Here's how the part is built. I have some questions about the finished solid (model axes, mm). A direction names the side the tool comes from. Coordinates: 2 decimals unless noted, no trailing zeros. Write each loop counter-clockwise with the first axis right and the second up, starting at its lowest first coordinate (ties: lowest second). Pieces come first, ordered by that corner, then holes.
```python
from build123d import *

# Parameters (mm, degrees)
SKETCH1_R           = 4.25
BOSS_EXTRUDE1_DEPTH = 20
SKETCH3_R           = 3.55
CUT_EXTRUDE2_DEPTH  = 10.5
SKETCH2_R           = 3.2
CUT_EXTRUDE3_DEPTH  = 10.5


with BuildPart() as part:
    # Sketch1 → Boss-Extrude1 (new body)
    with BuildSketch(Plane(origin=(0, 0, 0), x_dir=(1, 0, 0), z_dir=(0, 1, 0))):
        Polygon((0, 0), (0, 50), (57.5, 50), (72.5, 30), (87.5, 50), (145, 50), (145, 0), align=None)
        with Locations(Location((15, 20.25, 0), (0, 0, 270))):
            Circle(SKETCH1_R, mode=Mode.SUBTRACT)
        with Locations(Location((72.5, 14.25, 0), (0, 0, 270))):
            Circle(SKETCH1_R, mode=Mode.SUBTRACT)
        with Locations(Location((130, 20.25, 0), (0, 0, 270))):
            Circle(SKETCH1_R, mode=Mode.SUBTRACT)
    extrude(amount=BOSS_EXTRUDE1_DEPTH)

    # Sketch3 → Cut-Extrude2 (cut)
    with BuildSketch(Plane.XY):
        with Locations((25, 10)):
            Circle(SKETCH3_R)
        with Locations((120, 10)):
            Circle(SKETCH3_R)
    extrude(amount=-CUT_EXTRUDE2_DEPTH, mode=Mode.SUBTRACT)

    # Sketch2 → Cut-Extrude3 (cut)
    with BuildSketch(Plane(origin=(0, 20, 0), x_dir=(1, 0, 0), z_dir=(0, 1, 0))):
        with Locations(Location((22.5, 35, 0), (0, 0, 270))):
            Circle(SKETCH2_R)
        with Locations(Location((122.5, 35, 0), (0, 0, 270))):
            Circle(SKETCH2_R)
    extrude(amount=-CUT_EXTRUDE3_DEPTH, mode=Mode.SUBTRACT)


solid = part.part
```
1) Imagine slicing it at C-C on y = 2. Please give me the cut outline in (x, z), then the cut area to 3 significant figures.
Values follow:
outline: (0, -50) - (57.5, -50) - (72.5, -30) - (87.5, -50) - (145, -50) - (145, 0) - (0, 0) - close; hole circle Ø8.5 at (15, -20.25); hole circle Ø8.5 at (72.5, -14.25); hole circle Ø8.5 at (130, -20.25)
area: 6,780 mm2
2) We'd pull the mould along X, two halves only. Please class faces 1 (the face through (74, 10, 0)), 2 (the face through (120, 10, -10.5)), 3 (the face through (0, 10, -25)): pulls with the +X half, pulls with the -X half, needs draft (parallel to the pull), parting line crosses it, or undercut.
Values follow:
face 1: needs draft
face 2: undercut
face 3: pulls with the -X half
3) Imagine slicing it at A-A on x = 15. Please give me the cut outline in (y, z).
Values follow:
outline: (0, -50) - (20, -50) - (20, -24.5) - (0, -24.5) - close; (0, -16) - (20, -16) - (20, 0) - (0, 0) - close
4) Imagine slicing it at D-D on y = 16.25. Please give me the cut outline in (x, z).
Values follow:
outline: (0, -50) - (57.5, -50) - (72.5, -30) - (87.5, -50) - (145, -50) - (145, 0) - (0, 0) - close; hole circle Ø8.5 at (15, -20.25); hole circle Ø6.4 at (22.5, -35); hole circle Ø8.5 at (72.5, -14.25); hole circle Ø6.4 at (122.5, -35); hole circle Ø8.5 at (130, -20.25)
5) I need wall thicknesses on probe 1 along X at (y, z) = (7, -14.25); probe 2 along X at (y, z) = (17.5, -35); probe 3 along X at (y, z) = (7.5, -23). Which ranges of each line are inside material? Lowest first, please.
Values follow:
probe 1: x = 0 to 68.25, 76.75 to 145
probe 2: x = 0 to 19.3, 25.7 to 68.75, 76.25 to 119.3, 125.7 to 145
probe 3: x = 0 to 11.76, 18.24 to 126.76, 133.24 to 145
6) Imagine slicing it at B-B on z = -14.25. Please give me the cut outline in (x, y).
Values follow:
outline: (0, 0) - (68.25, 0) - (68.25, 20) - (0, 20) - close; (76.75, 0) - (145, 0) - (145, 20) - (76.75, 20) - close
7) Will these pins go through, and if not, where does the flat tip stop? pin 1 (4 mm diameter, centred on x = 73.5, y = 14, fed in from -Z); pin 2 (5 mm diameter, centred on x = 15, z = -20.25, fed in from -Y); pin 3 (1.9 mm diameter, centred on x = 23.5, z = -35.5, fed in from +Y); pin 4 (4.5 mm diameter, centred on x = 120, y = 10, fed in from +Z).
Values follow:
pin 1: stops at z = -34
pin 2: passes through
pin 3: stops at y = 9.5
pin 4: stops at z = -10.5
8) On a 3-axis mill with a long thin cutter (end or side, diameter ignored), from which of +Z, -Z, +X, -X, +Y, -Y can I reach the whole of each face in a straight line? I mean faces 4 (the face through (25, 10, -10.5)), 5 (the face through (74, 20, -25)), 6 (the face through (65, 10, -40)), 7 (the face through (25, 15, -37)), 8 (the face through (68.73, 9.86, -12.29)). Say none if no direction works.
Values follow:
face 4: +Z
face 5: +Z, -Z, +X, -X, +Y
face 6: -Z, +Y, -Y
face 7: +Y
face 8: +Y, -Y
